Part model, mm, in its own coordinate system. A direction names the side the tool comes from. Coordinates: 2 decimals unless noted, no trailing zeros. Write each loop counter-clockwise with the first axis right and the second up, starting at its lowest first coordinate (ties: lowest second). Pieces come first, ordered by that corner, then holes. Notation, with made-up numbers: (-8, -39) -> (33, -39) arc R16 cw to (33, -22) -> close; hole circle Ø10 at (-21, 11). An arc over 180 degrees is marked (long way). Write item = value, one per line.
from build123d import *

# Parameters (mm, degrees)
ESQUISSE1_W                                  = 12.6
ESQUISSE1_H                                  = 12.8
ESQUISSE1_R                                  = 1.65
BOSS_EXTRU_1_DEPTH                           = 5
BOSS_EXTRU_3_DEPTH                           = 6
BOSS_EXTRU_3_DEPTH_BACK                      = 5
ESQUISSE2_W                                  = 24.6
ESQUISSE2_H                                  = 2.5
FRAISAGE_POUR_VIS_T_TE_FRAIS_E_M2_51_A_COUNT = 2
FRAISAGE_POUR_VIS_T_TE_FRAIS_E_M2_51_A_PITCH = 18.6
CONG_3_R                                     = 0.5
ESQUISSE6_W                                  = 12.6
ESQUISSE6_H                                  = 3
BOSS_EXTRU_4_DEPTH                           = 10
ESQUISSE7_W                                  = 12.6
ESQUISSE7_H                                  = 5
BOSS_EXTRU_5_DEPTH                           = 5
ESQUISSE9_W                                  = 24.6
ESQUISSE9_H                                  = 2.538668555
BOSS_EXTRU_6_DEPTH                           = 3
ESQUISSE11_W                                 = 2
ESQUISSE11_H                                 = 8
BOSS_EXTRU_7_DEPTH                           = 25.3
CONG_4_R                                     = 1
CONG_5_R                                     = 1
CONG_6_R                                     = 1.5
CONG_7_R                                     = 1.5


with BuildPart() as part:
    # Esquisse1 → Boss.-Extru.1 (new body)
    with BuildSketch(Plane(origin=(0, 0, 0), x_dir=(1, 0, 0), z_dir=(0, 1, 0))):
        with Locations((0, -1.438202247)):
            Rectangle(ESQUISSE1_W, ESQUISSE1_H)
        with Locations(Location((0, 1.961797753, 0), (0, 0, 270))):
            Circle(ESQUISSE1_R, mode=Mode.SUBTRACT)
    extrude(amount=BOSS_EXTRU_1_DEPTH)

    # Esquisse2 → Boss.-Extru.3 (add, two sides: drawn at the far end of the back side and taken through both)
    with BuildSketch(Plane(origin=(0, 5, 0), x_dir=(1, 0, 0), z_dir=(0, 1, 0)).offset(-BOSS_EXTRU_3_DEPTH_BACK)):
        with Locations((0, -6.588202247)):
            Rectangle(ESQUISSE2_W, ESQUISSE2_H)
    extrude(amount=BOSS_EXTRU_3_DEPTH + BOSS_EXTRU_3_DEPTH_BACK)

    # Esquisse5 → Fraisage pour vis à tête fraisée M2.51 (revolve, cut)
    with BuildSketch(Plane(origin=(-9.3, 8, 5.338202247), x_dir=(0, 1, 0), z_dir=(1, 0, 0))):
        Polygon((0, 0), (0, 2.5), (1.475, 2.5), (1.45, 2.475), (1.45, 1.3), (2.75, 0), align=None)
    fraisage_pour_vis_t_te_frais_e_m2_51 = revolve(axis=Axis((-9.3, 8, -1.011797753), (0, 0, 1)), mode=Mode.SUBTRACT)

    # Fraisage pour vis à tête fraisée M2.51 a: Fraisage pour vis à tête fraisée M2.51 ×2
    with Locations(*[(i * FRAISAGE_POUR_VIS_T_TE_FRAIS_E_M2_51_A_PITCH, 0, 0) for i in range(1, FRAISAGE_POUR_VIS_T_TE_FRAIS_E_M2_51_A_COUNT)]):
        add(fraisage_pour_vis_t_te_frais_e_m2_51, mode=Mode.SUBTRACT)

    # Congé3
    cong_3_edges = [part.edges().sort_by_distance(p)[0] for p in [
        (0, 0, -3.611797753),
        (0, 5, -3.611797753),
    ]]
    fillet(cong_3_edges, radius=CONG_3_R)

    # Esquisse6 → Boss.-Extru.4 (add)
    with BuildSketch(Plane(origin=(0, 0, -4.961797753), x_dir=(-1, 0, 0), z_dir=(0, 0, -1))):
        with Locations((0, 3.5)):
            Rectangle(ESQUISSE6_W, ESQUISSE6_H)
    extrude(amount=BOSS_EXTRU_4_DEPTH)

    # Esquisse7 → Boss.-Extru.5 (add)
    with BuildSketch(Plane(origin=(0, 0, -14.961797753), x_dir=(-1, 0, 0), z_dir=(0, 0, -1))):
        with Locations((0, 2.5)):
            Rectangle(ESQUISSE7_W, ESQUISSE7_H)
    extrude(amount=BOSS_EXTRU_5_DEPTH)

    # Esquisse9 → Boss.-Extru.6 (add)
    with BuildSketch(Plane.XZ):
        with Locations((0, 6.607536525)):
            Rectangle(ESQUISSE9_W, ESQUISSE9_H)
    extrude(amount=BOSS_EXTRU_6_DEPTH)

    # Esquisse11 → Boss.-Extru.7 (add)
    with BuildSketch(Plane(origin=(0, 0, 5.338202247), x_dir=(-1, 0, 0), z_dir=(0, 0, -1))):
        with Locations((-7.3, 1)):
            Rectangle(ESQUISSE11_W, ESQUISSE11_H)
        with Locations((7.3, 1)):
            Rectangle(ESQUISSE11_W, ESQUISSE11_H)
    extrude(amount=BOSS_EXTRU_7_DEPTH)

    # Congé4
    cong_4_edges = [part.edges().sort_by_distance(p)[0] for p in [
        (0, 0, -14.961797753),
        (0, 2, -14.961797753),
        (0, 2, -4.961797753),
    ]]
    fillet(cong_4_edges, radius=CONG_4_R - 0.0001)  # a hair under: the kernel refuses the full size

    # Congé5
    cong_5_edges = [part.edges().sort_by_distance(p)[0] for p in [
        (6.3, -3, -7.311797753),
        (-6.3, -3, -7.311797753),
    ]]
    fillet(cong_5_edges, radius=CONG_5_R)

    # Congé6
    cong_6_edges = [part.edges().sort_by_distance(p)[0] for p in [
        (8.3, 5, -7.311797753),
        (-8.3, 5, -7.311797753),
    ]]
    fillet(cong_6_edges, radius=CONG_6_R)

    # Congé7
    cong_7_edges = [part.edges().sort_by_distance(p)[0] for p in [
        (-12.3, 11, 6.588202247),
        (12.3, 11, 6.588202247),
    ]]
    fillet(cong_7_edges, radius=CONG_7_R)


solid = part.part
Q1. Mould opens along Z. For faces 1 (the face through (-6.3, 0, -7)), 2 (the face through (0, 5, 7.838)), 3 (the face through (0, 5, -7)), 4 (the face through (6.3, 0, -7)) say: released by +Z, released by -Z, zero draft, split by the parting line, or undercut.
Model answer:
face_1 = undercut
face_2 = released by +Z
face_3 = zero draft
face_4 = undercut
Q2. Saw through at D-D on z = -7.25. Give the cut face in (x, y).
Model answer:
outline = (-8.3, -3) -> (-7.3, -3) arc R1 ccw to (-6.3, -2) -> (-6.3, 2) -> (6.3, 2) -> (6.3, -2) arc R1 ccw to (7.3, -3) -> (8.3, -3) -> (8.3, 3.5) arc R1.5 ccw to (6.8, 5) -> (-6.8, 5) arc R1.5 ccw to (-8.3, 3.5) -> close
Q3. Saw through at A-A on y = 8. Give the cut face in (x, z) (3 decimals).
Model answer:
outline = (-12.3, 5.338) -> (-12.05, 5.338) -> (-10.75, 6.638) -> (-10.75, 7.813) -> (-10.775, 7.838) -> (-12.3, 7.838) -> close; (-7.85, 6.638) -> (-6.55, 5.338) -> (6.55, 5.338) -> (7.85, 6.638) -> (7.85, 7.813) -> (7.825, 7.838) -> (-7.825, 7.838) -> (-7.85, 7.813) -> close; (10.75, 6.638) -> (12.05, 5.338) -> (12.3, 5.338) -> (12.3, 7.838) -> (10.775, 7.838) -> (10.75, 7.813) -> close
Q4. Probe line 1 (X direction, y = 8, z = 7); line 2 (X direction, y = -1.25, z = -15); line 3 (Y direction, x = -9.3, z = 6.95). List the from-to ranges inside material, lowest first. Write a range as from..to.
Model answer:
line_1 = -12.3..-10.75, -7.85..7.85, 10.75..12.3
line_2 = -8.3..-6.3, 6.3..8.3
line_3 = -3..6.55, 9.45..11
Q5. Which spindle directions (+Z, -Z, +X, -X, +Y, -Y) get a long thin tool onto all of the face, cutting with end or side? Do faces 5 (the face through (-7.85, 4.57, -7.49)), 6 (the face through (0, 2, -10)), 7 (the face through (-8.3, 0, -7)), 8 (the face through (-6.585, -2.699, -7.489)), 9 (the face through (0, 6, 5.338)). Say none if no direction does.
Model answer:
face_5 = -Z, -X, +Y
face_6 = -Y
face_7 = -Z, -X, +Y, -Y
face_8 = -Z, -Y
face_9 = -Z, +Y
Q6. Pin check, flat tips, straight feed: pin 1 (4 mm diameter, centred on x = -2, z = -12, fed in from +Y); pin 2 (1 mm diameter, centred on x = 1, y = 6, fed in from -Z); pin 3 (3 mm diameter, centred on y = -1, z = -1.5, fed in from +X). Stop position of each tip, or through.
Model answer:
pin_1 = 5
pin_2 = 5.34
pin_3 = 8.3
Q7. Saw through at C-C on y = 2.5. Give the cut face in (x, z).
Model answer:
outline = (-12.3, 5.34) -> (-8.3, 5.34) -> (-8.3, -19.96) -> (8.3, -19.96) -> (8.3, 5.34) -> (12.3, 5.34) -> (12.3, 7.84) -> (-12.3, 7.84) -> close; hole circle Ø3.3 at (0, -1.96)
Q8. Saw through at B-B on x = -9.3. Give the cut face in (y, z) (3 decimals), and give its area (3 significant figures).
Model answer:
outline = (-3, 5.338) -> (5.25, 5.338) -> (6.55, 6.638) -> (6.55, 7.813) -> (6.525, 7.838) -> (0, 7.838) -> (0, 7.877) -> (-3, 7.877) -> close; (9.45, 6.638) -> (10.75, 5.338) -> (11, 5.338) -> (11, 7.838) -> (9.475, 7.838) -> (9.45, 7.813) -> close
area = 26.2 mm²
